Design review of the part built by this model. Coordinates are the model's own, in mm. Give positions to 0.01 mm unless a question says otherwise; leave off trailing zeros. Write each loop counter-clockwise with the first axis right and the second up, starting at its lowest first coordinate (ties: lowest second). Pieces come first, ordered by that corner, then holes. Notation, with made-up numbers: M -4.5,20 L 1.5,20 A14 ccw 1.5,32 Z; hole C 15,50 d8. An arc over 180 degrees is marked long. Write each question's results on one line, items separated by ' | '. Start each with the question number.
from build123d import *

# Parameters (mm, degrees)
F0_R     = 4.3787819408
F0_R_2   = 2.76225
F1_DEPTH = 6.35


# Not quite as in the source:
# - a feature names something its author has since deleted; it is built from what else it names


with BuildPart() as f1:
    # F0 (on Front) → F1 (new body)
    with BuildSketch(Plane.XZ):
        with BuildLine():
            ThreePointArc((72.7984449517, 70.2034191426), (70.9385730123, 74.6935472031), (66.4484449517, 76.5534191426))
            Line((66.4484449517, 76.5534191426), (-66.6879298329, 76.5534191426))
            ThreePointArc((-66.6879298329, 76.5534191426), (-71.1780578935, 74.6935472031), (-73.0379298329, 70.2034191426))
            Line((-73.0379298329, 70.2034191426), (-73.0379298329, -14.1499808574))
            Line((-73.0379298329, -14.1499808574), (-73.0379298329, -42.5979808574))
            Line((-73.0379298329, -42.5979808574), (-73.0379298329, -56.7965808574))
            ThreePointArc((-73.0379298329, -56.7965808574), (-71.1780578935, -61.286708918), (-66.6879298329, -63.1465808574))
            Line((-66.6879298329, -63.1465808574), (67.2946030807, -63.1465808574))
            ThreePointArc((67.2946030807, -63.1465808574), (71.7847311412, -61.286708918), (73.6446030807, -56.7965808574))
            Line((73.6446030807, -56.7965808574), (73.6446030807, -42.5853939971))
            Line((73.6446030807, -42.5853939971), (72.7984449517, -14.1499808574))
            Line((72.7984449517, -14.1499808574), (72.7984449517, 70.2034191426))
        make_face()
        with Locations((-63.8573840261, -54.3791967528)):
            Circle(F0_R, mode=Mode.SUBTRACT)
        with Locations((-43.1257002056, -36.0373866536)):
            Circle(F0_R, mode=Mode.SUBTRACT)
        with Locations((0, -36.0373866536)):
            Circle(F0_R_2, mode=Mode.SUBTRACT)
        with Locations((-43.1257002056, 0)):
            Circle(F0_R, mode=Mode.SUBTRACT)
        Circle(F0_R_2, mode=Mode.SUBTRACT)
        with Locations((64.2901332332, -54.3791967528)):
            Circle(F0_R, mode=Mode.SUBTRACT)
        with Locations((41.3103699684, -36.0373866536)):
            Circle(F0_R_2, mode=Mode.SUBTRACT)
        with Locations((41.3103699684, 0)):
            Circle(F0_R_2, mode=Mode.SUBTRACT)
        with Locations((-43.1257002056, 36.3284125924)):
            Circle(F0_R, mode=Mode.SUBTRACT)
        with Locations((0, 36.3284125924)):
            Circle(F0_R_2, mode=Mode.SUBTRACT)
        with Locations((-63.8573840261, 70.3177154064)):
            Circle(F0_R, mode=Mode.SUBTRACT)
        with Locations((-21.2588757277, 70.3177154064)):
            Circle(F0_R_2, mode=Mode.SUBTRACT)
        with Locations((41.5558456844, 36.3284125924)):
            Circle(F0_R_2, mode=Mode.SUBTRACT)
        with Locations((20.5344017595, 70.3177154064)):
            Circle(F0_R_2, mode=Mode.SUBTRACT)
        with Locations((64.2901332332, 70.3177154064)):
            Circle(F0_R, mode=Mode.SUBTRACT)
    extrude(amount=F1_DEPTH)


solid = f1.part
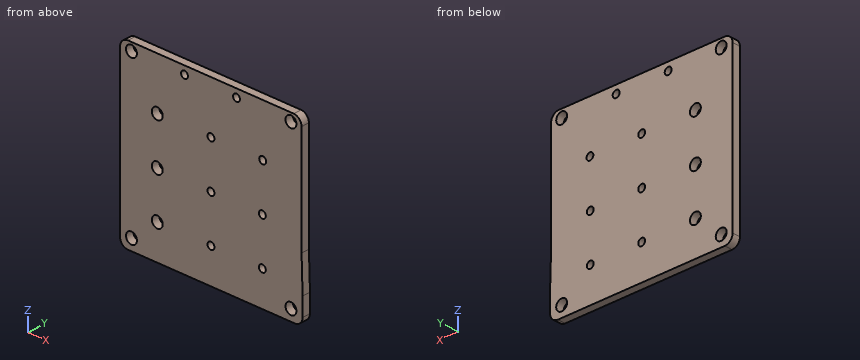
Q1. We need section B-B on z = 0. Write out the cut boundary in (x, y), and give its area (3 significant figures).
Q2. For pin 1 Ø5 at (x, z) = (-21.26, 70.32) entering from -Y, flat-tipped, find the tip position at first contact; note if it passes through.
Q3. We need section D-D on x = -20.5. Write out the cut boundary in (y, z).
Q4. We need section A-A on x = 0. Write out the cut boundary in (y, z), and give its area (3 significant figures).
Q5. We need section C-C on y = -2. Count the separate pieces of the cut face and the enclosed holes in it, and give its area (3 significant figures).
Q6. Wall thickness on line 1 along X through (y, z) = (-1.5, 37); line 2 along X through (y, z) = (-3, -52); line 3 along X through (y, z) = (-1.25, 35): over which ranges is each line inside the solid? List them lowest first. Write a range as from..to.
Answer sheet:
1) outline: M -73.04,-6.35 L -47.5,-6.35 L -47.5,0 L -73.04,0 Z; M -38.75,-6.35 L -2.76,-6.35 L -2.76,0 L -38.75,0 Z; M 2.76,-6.35 L 38.55,-6.35 L 38.55,0 L 2.76,0 Z; M 44.07,-6.35 L 72.8,-6.35 L 72.8,0 L 44.07,0 Z | area: 800 mm^2
2) pin 1: through
3) outline: M -6.35,-63.15 L 0,-63.15 L 0,67.66 L -6.35,67.66 Z; M -6.35,72.97 L 0,72.97 L 0,76.55 L -6.35,76.55 Z
4) outline: M -6.35,-63.15 L 0,-63.15 L 0,-38.8 L -6.35,-38.8 Z; M -6.35,-33.28 L 0,-33.28 L 0,-2.76 L -6.35,-2.76 Z; M -6.35,2.76 L 0,2.76 L 0,33.57 L -6.35,33.57 Z; M -6.35,39.09 L 0,39.09 L 0,76.55 L -6.35,76.55 Z | area: 782 mm^2
5) separate pieces: 1 | enclosed holes: 15 | area: 19,800 mm^2
6) line 1: -73.04..-47.45, -38.8..-2.68, 2.68..38.88, 44.24..72.8 | line 2: -73.04..-67.53, -60.18..60.61, 67.97..73.64 | line 3: -73.04..-47.3, -38.95..-2.42, 2.42..39.13, 43.98..72.8
